from build123d import *

# Parameters (mm, degrees)
F0_R     = 4.5
F0_R_2   = 5.5
F1_DEPTH = 15


with BuildPart() as f1:
    # F0 (on Right) → F1 (new body)
    with BuildSketch(Plane.YZ):
        with BuildLine():
            Line((-166.539142, 155), (-250, 155))
            Line((-250, 155), (-250, -185))
            Line((-250, -185), (-140, -245))
            Line((-140, -245), (0, -245))
            Line((0, -245), (140, -245))
            Line((140, -245), (250, -185))
            Line((250, -185), (250, 155))
            Line((250, 155), (166.539142, 155))
            ThreePointArc((166.539142, 155), (152.745356, 150.850215), (143.530869, 139.778516))
            Line((143.530869, 139.778516), (76.644435, -17.601329))
            ThreePointArc((76.644435, -17.601329), (60.05836, -37.530386), (35.229544, -45))
            Line((35.229544, -45), (0, -45))
            Line((0, -45), (-35.229544, -45))
            ThreePointArc((-35.229544, -45), (-60.05836, -37.530386), (-76.644435, -17.601329))
            Line((-76.644435, -17.601329), (-143.530869, 139.778516))
            ThreePointArc((-143.530869, 139.778516), (-152.745356, 150.850215), (-166.539142, 155))
        make_face()
        with Locations((-205, 65)):
            Circle(F0_R, mode=Mode.SUBTRACT)
        with Locations((-180, 90)):
            Circle(F0_R_2, mode=Mode.SUBTRACT)
        with Locations((-180, 110)):
            Circle(F0_R_2, mode=Mode.SUBTRACT)
        with Locations((-180, 130)):
            Circle(F0_R_2, mode=Mode.SUBTRACT)
        with Locations((180, 90)):
            Circle(F0_R_2, mode=Mode.SUBTRACT)
        with Locations((205, 65)):
            Circle(F0_R, mode=Mode.SUBTRACT)
        with Locations((180, 110)):
            Circle(F0_R_2, mode=Mode.SUBTRACT)
        with Locations((180, 130)):
            Circle(F0_R_2, mode=Mode.SUBTRACT)
    extrude(amount=F1_DEPTH)


solid = f1.part
Can you work these out from the model? Positions are in its coordinate system, mm. A direction names the side the tool comes from. Coordinates: 2 decimals unless noted, no trailing zeros. Write each loop counter-clockwise with the first axis right and the second up, starting at its lowest first coordinate (ties: lowest second). Pieces come first, ordered by that corner, then holes. Notation, with made-up numbers: M 41,61 L 65,61 A27 ccw 65,90 Z; hole C 50.25,23.25 d9. An arc over 180 degrees is marked long. Use one line per item in the form item = value.
Q1. If we section it at D-D (y = 180): Write out the boundary of the cut face in (x, z).
Model answer:
outline = M 0,-223.18 L 15,-223.18 L 15,84.5 L 0,84.5 Z; M 0,95.5 L 15,95.5 L 15,104.5 L 0,104.5 Z; M 0,115.5 L 15,115.5 L 15,124.5 L 0,124.5 Z; M 0,135.5 L 15,135.5 L 15,155 L 0,155 Z
Q2. For faces 5 (the flat face through (7, -2, -245)), 6 (the flat face through (7.395, 110.556, 62.19)), which set-ups out of +Z, -Z, +X, -X, +Y, -Y let a thin tool reach every point of the face, with its end or its side?
Model answer:
face_5 = -Z, +X, -X, +Y, -Y
face_6 = +Z, +X, -X
Q3. If we section it at B-B (z = 5): Write out the boundary of the cut face in (x, y), then the cut area to 3 significant figures.
Model answer:
outline = M 0,-250 L 15,-250 L 15,-86.25 L 0,-86.25 Z; M 0,86.25 L 15,86.25 L 15,250 L 0,250 Z
area = 4,910 mm^2
Q4. If we section it at C-C (z = 110): Write out the boundary of the cut face in (x, y) (3 decimals).
Model answer:
outline = M 0,-250 L 15,-250 L 15,-185.5 L 0,-185.5 Z; M 0,-174.5 L 15,-174.5 L 15,-130.875 L 0,-130.875 Z; M 0,130.875 L 15,130.875 L 15,174.5 L 0,174.5 Z; M 0,185.5 L 15,185.5 L 15,250 L 0,250 Z
Q5. If we section it at A-A (x = 12): State how many separate pieces and enclosed holes the cut face has, then the cut area to 3 significant figures.
Model answer:
separate_pieces = 1
enclosed_holes = 8
area = 150,000 mm^2
Q6. I need wall thicknesses on line 1 along Z through (x, y) = (6.75, 180); line 2 along Z through (x, y) = (5.25, -205); line 3 along Y through (x, z) = (4.25, 129.5). Which ranges of each line are inside material? Lowest first, please. Write a range as from..to.
Model answer:
line_1 = -223.18..84.5, 95.5..104.5, 115.5..124.5, 135.5..155
line_2 = -209.55..60.5, 69.5..155
line_3 = -250..-185.48, -174.52..-139.16, 139.16..174.52, 185.48..250
Q7. For P1, Ø4.5, axis at x = 4, y = -5, coming from the +Z side; P2, Ø6, axis at x = 5, y = 78, coming from the +Z side; P3, Ø2, axis at x = 3.5, z = -198.5, coming from the +Y side, each with a flat end and sliding along its axis, tell me the tip position at first contact or that it passes through.
Model answer:
P1 = -45
P2 = -7.35
P3 = 227.08
Q8. We'd pull the mould along Y, two halves only. Please class faces 1 (the flat face through (7.4, -195.77, -214.58)), 2 (the flat face through (7, 250, -17)), 3 (the cylindrical face through (7.4, -152.58, 150.74)), 4 (the flat face through (7, -208, 155)): +Y half, -Y half, draft (parallel to the pull), parting line (faces both ways), or undercut.
Model answer:
face_1 = -Y half
face_2 = +Y half
face_3 = undercut
face_4 = draft
